Geometry check sheet. Reference: drawing and pictorial views, mm from the part's lowest x, y, z. Give positions to 0.01 mm unless a question says otherwise; leave off trailing zeros. Loops run counter-clockwise (first coordinate to the right, second up) from the corner with the lowest first, then second, coordinate; pieces in that order, holes last. Notation, with made-up numbers: M -14,29.25 L 31,29.25 A29 cw 31,53.25 Z; hole C 30,20 d2. An arc over 180 degrees is marked long. Use CSV: the item, a comma, the result in double quotes.
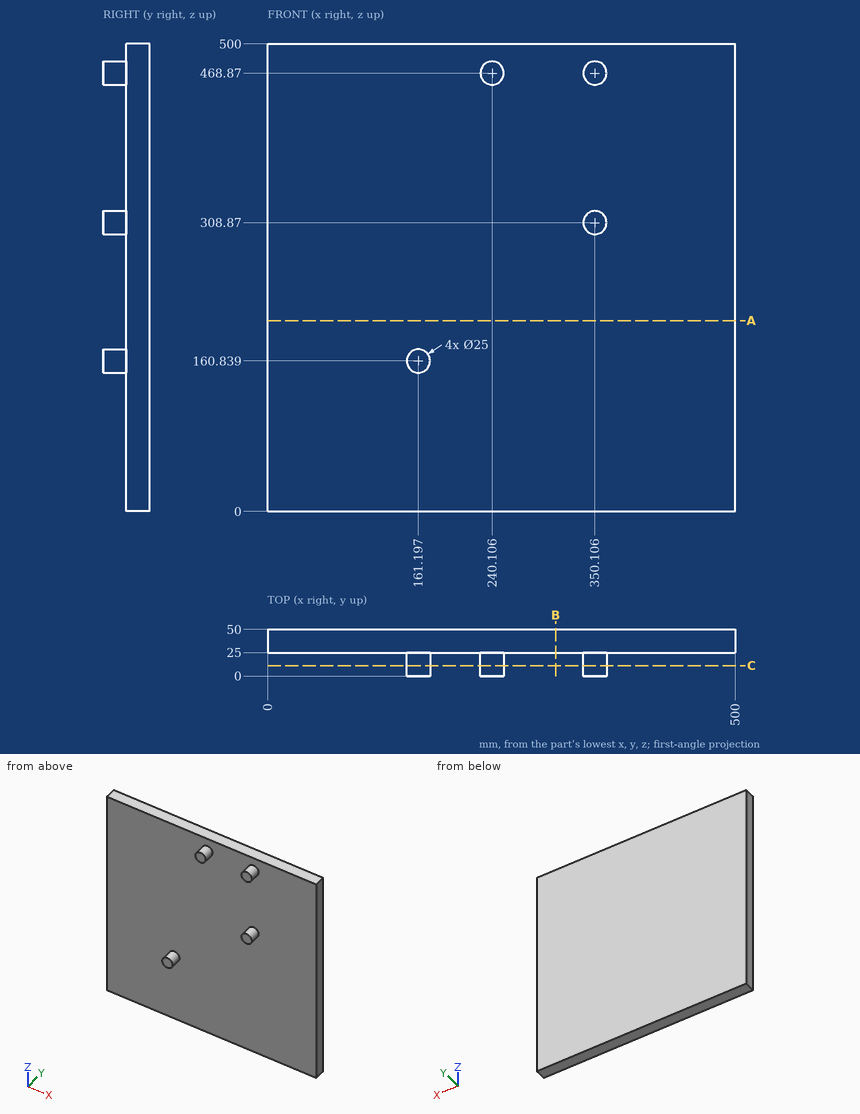
(1) Depth check by flat-ended pin: pin 1 Ø2 at (x, y) = (191.5, 25) entering from -Z. Enter the tip coordinate at first touch or a pass-through.
Calculated:
pin 1,"stops at z = 0"
(2) Scan lines: L1, parallel to Y at x = 368, z = 257.5; L2, parallel to X at y = 24.5, z = 159.5 (1 decimal); L3, parallel to X at y = 10, z = 465.5. Record each from-to range of solid material in increasing order. Write a range as from..to.
Calculated:
L1,"y = 25..50"
L2,"x = 148.8..173.6"
L3,"x = 228.07..252.14, 338.07..362.14"
(3) Section check C-C on y = 11. Record the cut outline in (x, z) (1 decimal), plus the area to 3 significant figures.
Calculated:
outline,"C 161.2,160.8 d25; C 240.1,468.9 d25; C 350.1,308.9 d25; C 350.1,468.9 d25"
area,"1,960 mm²"
(4) Section check B-B on x = 308. Record the cut outline in (y, z).
Calculated:
outline,"M 25,0 L 50,0 L 50,500 L 25,500 Z"
(5) Section check A-A on z = 204. Record the cut outline in (x, y).
Calculated:
outline,"M 0,25 L 500,25 L 500,50 L 0,50 Z"
